from build123d import *

# Parameters (mm, degrees)
EXTRUDE1_DEPTH            = 25.4
F_4_40_TAPPED_HOLE1_D     = 2.2606
F_4_40_TAPPED_HOLE1_DEPTH = 7.62
F_4_40_TAPPED_HOLE1_TIP   = 0.679152758
SKETCH5_R                 = 1.5875
EXTRUDE2_DEPTH            = 5.08


with BuildPart() as part:
    # Sketch1 → Extrude1 (new body)
    with BuildSketch(Plane(origin=(0, 0, 0), x_dir=(1, 0, 0), z_dir=(0, 1, 0))):
        Polygon((-1.374815329, 2.38125), (1.374815329, 2.38125), (2.749630657, 0), (1.374815329, -2.38125), (-1.374815329, -2.38125), (-2.749630657, 0), align=None)
    extrude(amount=EXTRUDE1_DEPTH)

    # #4-40 Tapped Hole1
    with Locations(Plane.ZX.offset(25.4)):
        with Locations((0, 0)):
            Hole(F_4_40_TAPPED_HOLE1_D / 2, depth=F_4_40_TAPPED_HOLE1_DEPTH)
            with Locations((0, 0, -(F_4_40_TAPPED_HOLE1_DEPTH + F_4_40_TAPPED_HOLE1_TIP / 2))):  # 118° drill point
                Cone(0, F_4_40_TAPPED_HOLE1_D / 2, F_4_40_TAPPED_HOLE1_TIP, mode=Mode.SUBTRACT)

    # Sketch5 → Extrude2 (add)
    with BuildSketch(Plane.XZ):
        Circle(SKETCH5_R)
    extrude(amount=EXTRUDE2_DEPTH)


solid = part.part
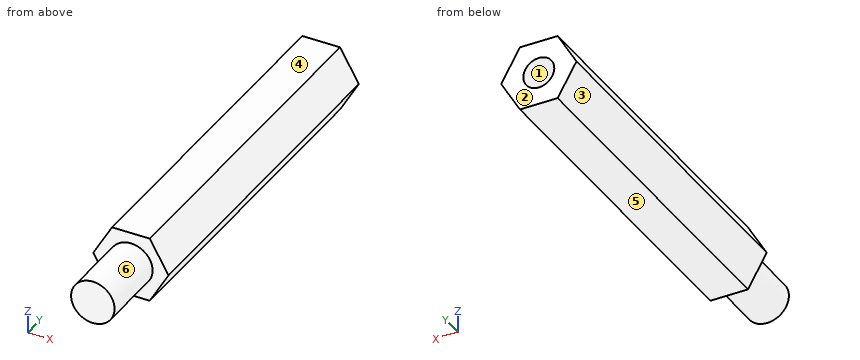
Could you check a few things on this model? Use its own coordinates, in mm. Face numbers are marked on the shaded views. A direction names the side the tool comes from. Give positions to 0.01 mm unless a question says otherwise; leave off trailing zeros. Order: outer loops, then holes, each group sorted by start corner. A loop starts at its lowest first (then second) coordinate and runs counter-clockwise, first axis right, second up. Notation, with made-up numbers: (25.25, 34.25) - (68.25, 34.25) arc R22 ccw to (68.25, 57.25) - close; hole circle Ø11 at (67.5, 54.5). An arc over 180 degrees is marked (long way). One line per question, with ' | ' between items. Start each with the question number.
Item 1: Thinking about a two-plate mould opening in Z: for the marked faces 1, 2, 3 and 4, which applies, pulls with the +Z half, pulls with the -Z half, needs draft (parallel to the pull), parting line crosses it, or undercut?
Item 2: For the marked faces 5 and 6, which set-ups out of +Z, -Z, +X, -X, +Y, -Y let a thin tool reach every point of the face, with its end or its side?
Item 3: I want a section at A-A on y = 4.5. Write out the boundary of the cut face in (x, z), then the cut area to 3 significant figures.
Item 4: I'm going to push a flat-ended pin straight in: pin 1 Ø1.8 at (x, z) = (0, 0) entering from +Y. Where does the tip first touch, or does it pass through?
Item 5: I need wall thicknesses on probe 1 along Z at (x, y) = (0, 23); probe 2 along Y at (x, z) = (0.4, 1.65); probe 3 along X at (y, z) = (13.5, 0.7). Which ranges of each line are inside material? Lowest first, please. Write a range as [from, to].
Verdict:
1) face 1: undercut | face 2: needs draft | face 3: pulls with the -Z half | face 4: pulls with the +Z half
2) face 5: -Z, +X, -X, +Y, -Y | face 6: -Y
3) outline: (-2.75, 0) - (-1.37, -2.38) - (1.37, -2.38) - (2.75, 0) - (1.37, 2.38) - (-1.37, 2.38) - close | area: 19.6 mm^2
4) pin 1: y = 17.64
5) probe 1: [-2.38, -1.13], [1.13, 2.38] | probe 2: [0, 25.4] | probe 3: [-2.35, 2.35]
